Check sheet for the modelled part. Datum: model origin and axes. Units: mm. Face numbers are marked on the shaded views. A direction names the side the tool comes from. Give positions to 0.01 mm unless a question says otherwise; leave off trailing zeros. Order: outer loops, then holes, each group sorted by start corner. A loop starts at its lowest first (then second) coordinate and runs counter-clockwise, first axis right, second up.
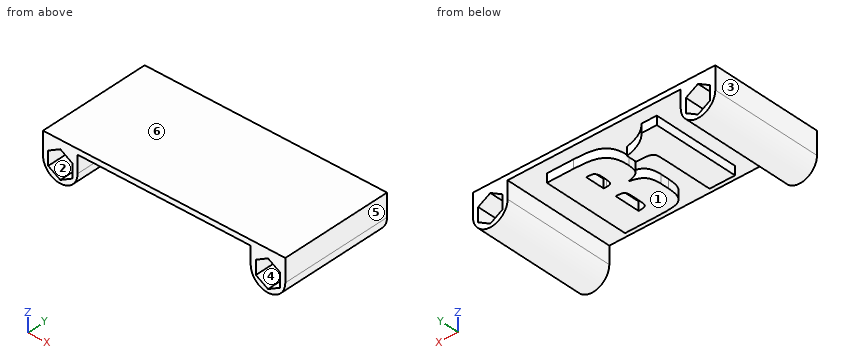
from build123d import *

# Parameters (mm, degrees)
BOSS_EXTRUDE1_DEPTH = 26
BOSS_EXTRUDE2_DEPTH = 2


with BuildPart() as part:
    # Sketch1 → Boss-Extrude1 (new body)
    with BuildSketch(Plane(origin=(0, 0, 0), x_dir=(1, 0, 0), z_dir=(0, 1, 0))):
        with BuildLine():
            Line((-28, 0), (-28, -5.233161507))
            Line((-28, -5.233161507), (28, -5.233161507))
            Line((28, -5.233161507), (28, 0))
            ThreePointArc((28, 0), (24, 4), (20, 0))
            Line((20, 0), (20, -4))
            Line((20, -4), (-20, -4))
            Line((-20, -4), (-20, 0))
            ThreePointArc((-20, 0), (-24, 4), (-28, 0))
        make_face()
        Polygon((-24, -3.233161507), (-21.2, -1.616580754), (-21.2, 1.616580754), (-24, 3.233161507), (-26.8, 1.616580754), (-26.8, -1.616580754), align=None, mode=Mode.SUBTRACT)
        Polygon((24, -3.233161507), (26.8, -1.616580754), (26.8, 1.616580754), (24, 3.233161507), (21.2, 1.616580754), (21.2, -1.616580754), align=None, mode=Mode.SUBTRACT)
    extrude(amount=BOSS_EXTRUDE1_DEPTH)

    # Sketch2 → Boss-Extrude2 (add)
    # profile 1 of 2: a face of its own
    with BuildSketch(Plane(origin=(0, 0, 4), x_dir=(-1, 0, 0), z_dir=(0, 0, -1))):
        with BuildLine():
            Line((-13.647058824, 23), (-7.511029412, 23))
            add(Edge.make_bspline(
                [(-7.511029412, 23), (-7.275731179, 22.997981779), (-6.819798363, 22.994071112), (-6.159048704, 22.98133809), (-5.542304381, 22.952753821), (-4.97019879, 22.906571513), (-4.43999705, 22.85840676), (-3.95570662, 22.791983867), (-3.515425024, 22.714754032), (-3.113311884, 22.62754473), (-2.741946911, 22.520639825), (-2.392633853, 22.391003364), (-2.061356263, 22.237036075), (-1.749186518, 22.056973854), (-1.455538155, 21.852418481), (-1.180448032, 21.624572715), (-0.921358069, 21.373380515), (-0.680179003, 21.096140802), (-0.459212321, 20.785039798), (-0.272594718, 20.428388227), (-0.114539747, 20.02893381), (0.01166681, 19.585017574), (0.11595967, 19.100276176), (0.182028181, 18.570062266), (0.228008391, 17.997136115), (0.232808413, 17.599367786), (0.235294118, 17.393382353)],
                knots=[0, 0, 0, 0, 1.509097582, 2.924149082, 4.238183516, 5.467880876, 6.60497888, 7.652028453, 8.60175528, 9.471282623, 10.289610236, 11.077949411, 11.85853237, 12.62964082, 13.386192643, 14.150986854, 14.917998976, 15.698027796, 16.504800181, 17.359170498, 18.272796439, 19.255228546, 20.31576025, 21.449539682, 22.679237042, 24, 24, 24, 24], degree=3))
            add(Edge.make_bspline(
                [(0.235294118, 17.393382353), (0.232974752, 17.254856933), (0.228515198, 16.98850749), (0.200383988, 16.605202315), (0.149069438, 16.255170164), (0.079129695, 15.936955638), (-0.005906464, 15.649717168), (-0.117746792, 15.395642258), (-0.249513114, 15.174191871), (-0.404256499, 14.979905609), (-0.591024507, 14.809913361), (-0.814712612, 14.657824833), (-1.072004992, 14.508015165), (-1.37363652, 14.380830632), (-1.707083821, 14.248019836), (-2.08498403, 14.138316996), (-2.498813667, 14.030114219), (-2.790094496, 13.971551743), (-2.941176471, 13.941176471)],
                knots=[0, 0, 0, 0, 1.248797497, 2.401122606, 3.461961877, 4.434949853, 5.336516199, 6.157599865, 6.930603047, 7.653512509, 8.388476874, 9.197582017, 10.088252902, 11.067492471, 12.144601044, 13.32232985, 14.611142055, 16, 16, 16, 16], degree=3))
            add(Edge.make_bspline(
                [(-2.941176471, 13.941176471), (-2.770371191, 13.906426369), (-2.441331923, 13.839483779), (-1.972356815, 13.710080705), (-1.546384653, 13.563684789), (-1.161438092, 13.403562089), (-0.820288891, 13.222788974), (-0.522021254, 13.024823635), (-0.263588432, 12.811780764), (-0.05097915, 12.573648761), (0.133439784, 12.315749283), (0.287925528, 12.026254146), (0.414834382, 11.704673071), (0.522237978, 11.351932642), (0.605600404, 10.96831546), (0.663113943, 10.5516397), (0.701055467, 10.10487322), (0.704241313, 9.795426457), (0.705882353, 9.636029412)],
                knots=[0, 0, 0, 0, 1.318474424, 2.539908949, 3.677602242, 4.724633259, 5.691096321, 6.593718157, 7.429479115, 8.217211742, 9.001882654, 9.823273564, 10.69276163, 11.613722017, 12.610358031, 13.659357769, 14.794327495, 16, 16, 16, 16], degree=3))
            Line((0.705882353, 9.636029412), (0.705882353, 7.757352941))
            add(Edge.make_bspline(
                [(0.705882353, 7.757352941), (0.704799402, 7.591884318), (0.702704249, 7.27175714), (0.67738761, 6.807934298), (0.632072604, 6.377720507), (0.577490967, 5.978821137), (0.492846489, 5.615803116), (0.405671971, 5.281599354), (0.28994872, 4.983831187), (0.160842329, 4.715033057), (0.012977275, 4.472562188), (-0.158442094, 4.255363641), (-0.345211479, 4.055514692), (-0.555509379, 3.876624389), (-0.785166734, 3.715553429), (-1.037562672, 3.576418256), (-1.307049122, 3.453168174), (-1.607705683, 3.35203056), (-1.957946085, 3.265715552), (-2.377158841, 3.195476641), (-2.873785211, 3.13277364), (-3.4493738, 3.088655391), (-4.103756338, 3.047411202), (-4.83799783, 3.018157261), (-5.650694295, 3.005897294), (-6.218135233, 3.002024237), (-6.514705882, 3)],
                knots=[0, 0, 0, 0, 1.152396282, 2.229506502, 3.233379135, 4.165256051, 5.030866667, 5.828132484, 6.56839727, 7.251703786, 7.90313474, 8.541689401, 9.175664088, 9.805199082, 10.461088127, 11.125968039, 11.809754162, 12.52233939, 13.331757138, 14.319645788, 15.481015661, 16.817142782, 18.339330194, 20.047761731, 21.934379081, 24, 24, 24, 24], degree=3))
            Line((-6.514705882, 3), (-13.647058824, 3))
            Line((-13.647058824, 3), (-13.647058824, 23))
        make_face()
        with BuildLine():
            Line((-7.529411765, 19.705882353), (-7.529411765, 15.235294118))
            add(Edge.make_bspline(
                [(-7.529411765, 15.235294118), (-7.406866635, 15.237978484), (-7.192422866, 15.242675901), (-6.977943364, 15.24522929), (-6.886029412, 15.246323529)],
                knots=[0, 0, 0, 0, 1.142911548, 2, 2, 2, 2], degree=3))
            add(Edge.make_bspline(
                [(-6.886029412, 15.246323529), (-6.740947301, 15.248687273), (-6.477856737, 15.252973663), (-6.125517198, 15.325927539), (-5.851081785, 15.437107788), (-5.684278021, 15.590100017), (-5.601180942, 15.752298454), (-5.553614641, 15.915978468), (-5.509206909, 16.121100191), (-5.474341123, 16.370628298), (-5.445721739, 16.665000056), (-5.423400941, 17.002143802), (-5.413861666, 17.38352185), (-5.412490731, 17.651958103), (-5.411764706, 17.794117647)],
                knots=[0, 0, 0, 0, 1.48265011, 2.688624062, 3.665886862, 4.482415445, 4.937118978, 5.516533753, 6.222944153, 7.08542788, 8.094324435, 9.251250026, 10.544306002, 12, 12, 12, 12], degree=3))
            add(Edge.make_bspline(
                [(-5.411764706, 17.794117647), (-5.414328018, 17.940093199), (-5.419057143, 18.209407536), (-5.458346473, 18.577258961), (-5.518349704, 18.87773136), (-5.617120488, 19.109882781), (-5.733904141, 19.290128296), (-5.868891145, 19.428124069), (-6.017897311, 19.536117272), (-6.198796129, 19.605125943), (-6.426159943, 19.646746329), (-6.722318383, 19.677870943), (-7.099011903, 19.698357172), (-7.37742421, 19.703224978), (-7.529411765, 19.705882353)],
                knots=[0, 0, 0, 0, 1.519775244, 2.803875429, 3.850524394, 4.696904465, 5.415553468, 6.074478191, 6.697696669, 7.316323432, 8.072315065, 9.09987747, 10.416799398, 12, 12, 12, 12], degree=3))
        make_face(mode=Mode.SUBTRACT)
        with BuildLine():
            Line((-7.529411765, 12.176470588), (-7.529411765, 6.294117647))
            add(Edge.make_bspline(
                [(-7.529411765, 6.294117647), (-7.420324785, 6.298478074), (-7.213005859, 6.306765029), (-6.918337489, 6.326902982), (-6.654951975, 6.361663585), (-6.420932841, 6.399065544), (-6.218252281, 6.450542123), (-6.047062066, 6.509147737), (-5.904616172, 6.57395291), (-5.788177353, 6.653131279), (-5.695063658, 6.755503737), (-5.618691129, 6.883359348), (-5.55127953, 7.03989887), (-5.504628482, 7.228008812), (-5.457915355, 7.44189207), (-5.430019896, 7.68684309), (-5.417623422, 7.96064691), (-5.413774101, 8.153174564), (-5.411764706, 8.253676471)],
                knots=[0, 0, 0, 0, 1.50566656, 2.861507154, 4.071047619, 5.168542278, 6.12771314, 6.950823291, 7.661450358, 8.28034255, 8.878344747, 9.553732332, 10.32599646, 11.219809833, 12.220801373, 13.344401423, 14.613743465, 16, 16, 16, 16], degree=3))
            Line((-5.411764706, 8.253676471), (-5.411764706, 10.216911765))
            add(Edge.make_bspline(
                [(-5.411764706, 10.216911765), (-5.411625539, 10.323574104), (-5.411361354, 10.526054691), (-5.431934549, 10.812872087), (-5.455941272, 11.068312667), (-5.490634178, 11.28988458), (-5.538399387, 11.478501022), (-5.596797759, 11.632421229), (-5.660721533, 11.759017199), (-5.746931785, 11.854699599), (-5.860081356, 11.921764358), (-5.99584109, 11.985178234), (-6.168589838, 12.034357698), (-6.373799547, 12.077524186), (-6.614452953, 12.113799181), (-6.88926906, 12.14220067), (-7.198264679, 12.164205556), (-7.415407511, 12.172248096), (-7.529411765, 12.176470588)],
                knots=[0, 0, 0, 0, 1.448679605, 2.750075608, 3.904849468, 4.934080626, 5.79427915, 6.542621099, 7.168507459, 7.710604877, 8.264840309, 8.942819976, 9.743425019, 10.697014228, 11.792022656, 13.047885967, 14.450082115, 16, 16, 16, 16], degree=3))
        make_face(mode=Mode.SUBTRACT)
    # profile 2 of 2: a face of its own
    with BuildSketch(Plane(origin=(0, 0, 4), x_dir=(-1, 0, 0), z_dir=(0, 0, -1))):
        with BuildLine():
            Line((11.764705882, 23), (11.764705882, 3))
            Line((11.764705882, 3), (5.882352941, 3))
            Line((5.882352941, 3), (5.882352941, 13.639705882))
            add(Edge.make_bspline(
                [(5.882352941, 13.639705882), (5.880947737, 13.82230104), (5.878288215, 14.167884759), (5.877255074, 14.65816143), (5.865236193, 15.090768646), (5.851316968, 15.465840003), (5.833299033, 15.783338952), (5.812277963, 16.043366084), (5.787966916, 16.246039236), (5.751675327, 16.439313374), (5.671063802, 16.635997331), (5.513570677, 16.831585631), (5.300972739, 16.994325057), (5.081905966, 17.105669586), (4.863856573, 17.175428694), (4.65061388, 17.221357274), (4.394651874, 17.266432937), (4.092334468, 17.296767422), (3.746641909, 17.32251546), (3.355542137, 17.340185318), (2.920406806, 17.351060405), (2.615203504, 17.352296115), (2.455882353, 17.352941176)],
                knots=[0, 0, 0, 0, 1.706209308, 3.229210257, 4.580842603, 5.749723113, 6.736155842, 7.552061302, 8.186936249, 8.642816617, 9.387119351, 10.145384432, 10.960888028, 11.872433023, 12.426467721, 13.095924105, 13.909173589, 14.853778768, 15.933135423, 17.148271002, 18.511350491, 20, 20, 20, 20], degree=3))
            Line((2.455882353, 17.352941176), (1.882352941, 17.352941176))
            Line((1.882352941, 17.352941176), (1.882352941, 19.647058824))
            add(Edge.make_bspline(
                [(1.882352941, 19.647058824), (2.221677388, 19.719791453), (2.884869887, 19.861943704), (3.838958585, 20.14553208), (4.730122825, 20.484470888), (5.558298884, 20.876645002), (6.325128134, 21.323798016), (7.029371007, 21.823696326), (7.671429441, 22.379342308), (8.048042826, 22.79388857), (8.235294118, 23)],
                knots=[0, 0, 0, 0, 1.137311521, 2.22281794, 3.259150006, 4.260062448, 5.223308807, 6.165267245, 7.087775173, 8, 8, 8, 8], degree=3))
            Line((8.235294118, 23), (11.764705882, 23))
        make_face()
    extrude(amount=BOSS_EXTRUDE2_DEPTH)


solid = part.part
1) Section check C-C, the plane x = -23. Record the cut outline in (y, z).
Recorded:
outline: (0, -3.87) - (26, -3.87) - (26, -2.66) - (0, -2.66) - close; (0, 2.66) - (26, 2.66) - (26, 5.23) - (0, 5.23) - close
2) Depth check by flat-ended pin: pin 1 Ø0.6 at (x, y) = (6, 18.5) entering from -Z; pin 2 Ø0.5 at (x, z) = (-2, 3) entering from -Y; pin 3 Ø12 at (x, y) = (-17.5, 22.5) entering from -Z. Enter the tip coordinate at first touch or a pass-through.
Recorded:
pin 1: stops at z = 4
pin 2: stops at y = 17.35
pin 3: stops at z = -3.97
3) Set-up check for the marked faces 1, 2 and 3: record each of +Z, -Z, +X, -X, +Y, -Y from which the full face is reachable in a straight line by a thin tool's end or side.
Recorded:
face 1: -Z, +Y, -Y
face 2: +Y, -Y
face 3: +Z, -Z, -X, +Y, -Y
4) Section check A-A, the plane x = 22.5. Record the cut outline in (y, z), then the cut area to 3 significant figures.
Recorded:
outline: (0, -3.71) - (26, -3.71) - (26, -2.37) - (0, -2.37) - close; (0, 2.37) - (26, 2.37) - (26, 5.23) - (0, 5.23) - close
area: 109 mm2
5) Draft check along X on the marked faces 4, 5 and 6. Enter one of: +X half, -X half, draft (parallel to the pull), parting line (faces both ways), or undercut.
Recorded:
face 4: undercut
face 5: +X half
face 6: draft
6) Section check D-D, the plane y = 20.75. State how many separate pieces and enclosed holes the cut face has, then the cut area to 3 significant figures.
Recorded:
separate pieces: 1
enclosed holes: 2
area: 168 mm2
7) Material ranges on L1, parallel to X at y = 7.25, z = 1.5; L2, parallel to X at y = 17.75, z = -1; L3, parallel to Z at x = 15, y = 22, recorded low to high.
Recorded:
L1: x = -28 to -26.8, -21.2 to -20, 20 to 21.2, 26.8 to 28
L2: x = -27.87 to -26.8, -21.2 to -20.13, 20.13 to 21.2, 26.8 to 27.87
L3: z = 4 to 5.23
8) Section check B-B, the plane z = -2.5. Record the cut outline in (x, y).
Recorded:
outline: (-27.12, 0) - (-25.27, 0) - (-25.27, 26) - (-27.12, 26) - close; (-22.73, 0) - (-20.88, 0) - (-20.88, 26) - (-22.73, 26) - close; (20.88, 0) - (22.73, 0) - (22.73, 26) - (20.88, 26) - close; (25.27, 0) - (27.12, 0) - (27.12, 26) - (25.27, 26) - close
